```python
from build123d import *

# Parameters (mm, degrees)
CROQUIS1_W              = 12.7
CROQUIS1_H              = 25.4
SALIENTE_EXTRUIR1_DEPTH = 110
CROQUIS2_W              = 90
CROQUIS2_H              = 12.7
SALIENTE_EXTRUIR2_DEPTH = 12.7
CROQUIS3_R              = 3.5
CORTAR_EXTRUIR1_DEPTH   = 120.525269295
CROQUIS4_R              = 2.494853736
CROQUIS4_R_2            = 2.482276025
CORTAR_EXTRUIR2_DEPTH   = 81.244781762


with BuildPart() as part:
    # Croquis1 → Saliente-Extruir1 (new body)
    with BuildSketch(Plane(origin=(0, 0, 0), x_dir=(1, 0, 0), z_dir=(0, 1, 0))):
        Rectangle(CROQUIS1_W, CROQUIS1_H)
    extrude(amount=SALIENTE_EXTRUIR1_DEPTH)

    # Croquis2 → Saliente-Extruir2 (add)
    with BuildSketch(Plane(origin=(6.35, 0, 0), x_dir=(0, 0, -1), z_dir=(1, 0, 0))):
        with Locations((0, 40)):
            Rectangle(CROQUIS2_W, CROQUIS2_H)
    extrude(amount=SALIENTE_EXTRUIR2_DEPTH)

    # Croquis3 → Cortar-Extruir1 (cut, through all)
    with BuildSketch(Plane(origin=(6.35, 0, 0), x_dir=(0, 0, -1), z_dir=(1, 0, 0))):
        with Locations((0, 10)):
            Circle(CROQUIS3_R)
    extrude(amount=-CORTAR_EXTRUIR1_DEPTH, mode=Mode.SUBTRACT)

    # Croquis4 → Cortar-Extruir2 (cut, through all)
    with BuildSketch(Plane(origin=(0, 46.35, 0), x_dir=(1, 0, 0), z_dir=(0, 1, 0))):
        with Locations(Location((12.7, 35, 0), (0, 0, 270))):
            Circle(CROQUIS4_R)
        with Locations(Location((12.7, -35, 0), (0, 0, 270))):
            Circle(CROQUIS4_R_2)
    extrude(amount=-CORTAR_EXTRUIR2_DEPTH, mode=Mode.SUBTRACT)


solid = part.part
```
Check sheet for the modelled part. Datum: model origin and axes. Units: mm. A direction names the side the tool comes from. Give positions to 0.01 mm unless a question says otherwise; leave off trailing zeros. Write each loop counter-clockwise with the first axis right and the second up, starting at its lowest first coordinate (ties: lowest second). Pieces come first, ordered by that corner, then holes. Notation, with made-up numbers: (-15, -19) -> (28, -19) arc R12 ccw to (28, -9) -> close; hole circle Ø4 at (82, 87.5). An arc over 180 degrees is marked (long way). Use CSV: the item, a comma, the result in double quotes. Start each with the question number.
Q1. Cross-section at A-A on x = 12.7. Enter the section's corners in (y, z).
Q2. Release check for a two-part mould opening along Z. For faces 4 (the cylindrical face through (0.089, 6.583, 0.759)), 5 (the flat face through (13, 46.35, 1)), 6 (the flat face through (13, 40, 45)), 7 (the cylindrical face through (11.19, 40.09, 33.03)) record: +Z half, -Z half, draft (parallel to the pull), parting line (faces both ways), or undercut.
Q3. Scan lines: line 1 along X through (y, z) = (44.25, -35); line 2 along Y through (x, z) = (-3.75, 0); line 3 along Z through (x, y) = (-3.5, 47.5). Record each from-to range of solid material in increasing order.
Q4. Cross-section at D-D on y = 10. Enter the section's corners in (x, z), and give its area (3 significant figures).
Q5. Depth check by flat-ended pin: P1, Ø8, axis at x = 12.7, z = -35, coming from the -Y side; P2, Ø3, axis at x = 3.5, y = 98.5, coming from the +Z side; P3, Ø7.5, axis at y = 16.5, z = 0, coming from the +X side. Enter the tip coordinate at first touch or a pass-through.
Q6. Cross-section at B-B on z = 0. Enter the section's corners in (x, y), and give its area (3 significant figures).
Q7. Cross-section at C-C on y = 38.5. Enter the section's corners in (x, z), and give its area (3 significant figures).
Q8. Tool access check on faces 1 (the flat face through (6.35, 78, 0)), 2 (the flat face through (13, 33.65, 1)), 3 (the flat face through (6.35, 40, 29)). Record the directions out of +Z, -Z, +X, -X, +Y, -Y that give a thin tool (end or side, any length) a straight path to the whole face; none if there is none.
Working result:
1,outline,"(33.65, -45) -> (46.35, -45) -> (46.35, -37.49) -> (33.65, -37.49) -> close; (33.65, -32.51) -> (46.35, -32.51) -> (46.35, 32.52) -> (33.65, 32.52) -> close; (33.65, 37.48) -> (46.35, 37.48) -> (46.35, 45) -> (33.65, 45) -> close"
2,face 4,"undercut"
2,face 5,"draft"
2,face 6,"+Z half"
2,face 7,"undercut"
3,line 1,"x = 6.35 to 10.21, 15.19 to 19.05"
3,line 2,"y = 0 to 6.5, 13.5 to 110"
3,line 3,"z = -12.7 to 12.7"
4,outline,"(-6.35, -12.7) -> (6.35, -12.7) -> (6.35, -3.5) -> (-6.35, -3.5) -> close; (-6.35, 3.5) -> (6.35, 3.5) -> (6.35, 12.7) -> (-6.35, 12.7) -> close"
4,area,"234 mm^2"
5,P1,"stops at y = 33.65"
5,P2,"stops at z = 12.7"
5,P3,"stops at x = 6.35"
6,outline,"(-6.35, 0) -> (6.35, 0) -> (6.35, 6.5) -> (-6.35, 6.5) -> close; (-6.35, 13.5) -> (6.35, 13.5) -> (6.35, 33.65) -> (19.05, 33.65) -> (19.05, 46.35) -> (6.35, 46.35) -> (6.35, 110) -> (-6.35, 110) -> close"
6,area,"1,470 mm^2"
7,outline,"(-6.35, -12.7) -> (6.35, -12.7) -> (6.35, -45) -> (19.05, -45) -> (19.05, 45) -> (6.35, 45) -> (6.35, 12.7) -> (-6.35, 12.7) -> close; hole circle Ø4.99 at (12.7, -35); hole circle Ø4.96 at (12.7, 35)"
7,area,"1,430 mm^2"
8,face 1,"+Z, -Z, +X, +Y"
8,face 2,"+Z, -Z, +X, -Y"
8,face 3,"+Z, -X, +Y, -Y"
